Design review of the part shown in the three views and the two pictorial views. Dimensions are in mm from the part's minimum x, y and z. Coordinates: 2 decimals unless noted, no trailing zeros. Loops run counter-clockwise (first coordinate to the right, second up) from the corner with the lowest first, then second, coordinate; pieces in that order, holes last.
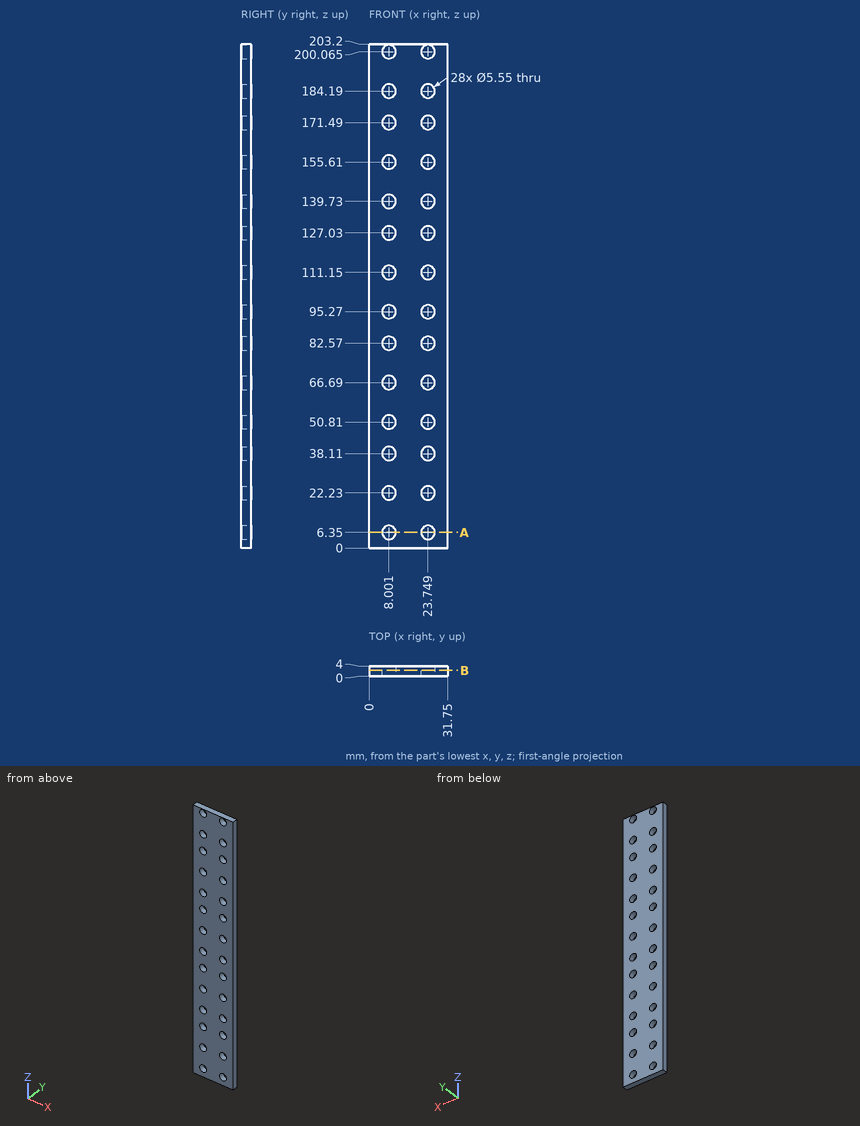
Q1. Consider section B-B (y = 2.25). Count the separate pieces of the cut face and the enclosed holes in it, then the cut area to 3 significant figures.
Q2. Consider section A-A (z = 6.35). State the section outline as (x, y) points, then the cut area to 3 significant figures.
Q3. For pin 1 Ø5 at (x, z) = (8.001, 6.35) entering from -Y, flat-tipped, find the tip position at first contact; note if it passes through.
Q4. Wall thickness on probe 1 along X at (y, z) = (2.5, 82.5); probe 2 along X at (y, z) = (3.35, 93): over which ranges is each line inside the solid? List them lowest first.
Model answer:
1. separate pieces: 1
1. enclosed holes: 28
1. area: 5,770 mm2
2. outline: (0, 0) - (5.23, 0) - (5.23, 4) - (0, 4) - close; (10.78, 0) - (20.97, 0) - (20.97, 4) - (10.78, 4) - close; (26.52, 0) - (31.75, 0) - (31.75, 4) - (26.52, 4) - close
2. area: 82.6 mm2
3. pin 1: passes through
4. probe 1: x = 0 to 5.23, 10.78 to 20.97, 26.52 to 31.75
4. probe 2: x = 0 to 6.4, 9.6 to 22.15, 25.35 to 31.75
